Geometry: final body of the model. Coordinates: model frame, mm. A direction names the side the tool comes from. Give positions to 0.01 mm unless a question says otherwise; leave off trailing zeros. Loops run counter-clockwise (first coordinate to the right, second up) from the corner with the lowest first, then second, coordinate; pieces in that order, holes last. Notation, with made-up numbers: (-31, 77.25) -> (18, 77.25) arc R29 cw to (18, 116.25) -> close; hole circle Ø8 at (77, 48.5). An arc over 180 degrees is marked (long way). One line per item, written item: value. Start each with the question number.
Autodesk Inventor part; units mm, degrees
ref_plane "XZ Plane" through (0, 0, 0) normal (0, 1, 0) x (-1, 0, 0)
ref_plane "XY Plane" through (0, 0, 0) normal (0, 0, 1) x (1, 0, 0)
sketch "Sketch1" plane through (0, 0, 0) normal (0, 0, 1) x (1, 0, 0)
  circle A0 centre (0, 0) radius 76.2
  dimension "tubeDiameter" = 152.4
extrude "Extrusion1" add sketch "Sketch1" along normal mid plane 438.15
sketch "Sketch2" plane through (0, 0, -219.075) normal (0, 0, -1) x (-1, 0, 0)
  circle A0 centre (0, 0) radius 69.85
  dimension "d6" = 139.7
extrude "Extrusion2" cut sketch "Sketch2" against normal blind 406.4
sketch "Sketch3" plane through (0, 0, 219.075) normal (0, 0, 1) x (1, 0, 0)
  circle A0 centre (0, 0) radius 82.55
  circle A1 centre (0, 0) radius 76.2
  dimension "d9" = 165.1
extrude "Extrusion3" add sketch "Sketch3" against normal blind 25.4
sketch "Sketch4" plane through (0, 0, -219.075) normal (0, 0, -1) x (-1, 0, 0)
  circle A0 centre (0, 0) radius 76.2
  circle A1 centre (0, 0) radius 82.55
extrude "Extrusion4" add sketch "Sketch4" against normal blind 25.4
properties part number "telescopeTube" material "Nylon, molybdenum disulphide"
Item 1: Mould query, pull axis X, two halves, no side actions, for faces 4 (the face through (1, 1, 187.325)), 5 (the face through (-60.47, -46.367, 2.711)), 6 (the face through (68, 19, -219.075)). Classes: pulls with the +X half, pulls with the -X half, needs draft (parallel to the pull), parting line crosses it, or undercut.
Item 2: Access query for faces 1 (the face through (-17.895, -80.587, 206.553)), 2 (the face through (-24, -73, -193.675)), 3 (the face through (55.431, -42.503, -18.72)). Directions: +Z, -Z, +X, -X, +Y, -Y. A direction counts if a zero-diameter tool reaches every point of the face in a straight line with its end or side. Return the directions, or none.
Item 3: Ray query, line 1 along Y through (x, z) = (0, 76); line 2 along Z through (x, y) = (54.5, 26.5) (3 decimals); line 3 along Y through (x, z) = (-50.5, 145). Return the intervals inside material, ascending. Write a range as [from, to].
Item 4: Section B-B, the plane y = -54. Output: boundary loops of the cut face in (x, z) (3 decimals), then the cut area to 3 significant figures.
Item 5: Pin query (flat end, axial travel): pin 1 (12 mm diameter, centred on x = -6.5, z = 33, fed in from +Y); pin 2 (1.5 mm diameter, centred on x = 47.5, z = -141, fed in from +Y); pin 3 (1 mm diameter, centred on x = 42.5, z = -132, fed in from -Y). Return the tip coordinate at first contact, or that it passes through.
Item 6: Section A-A, the plane x = 0. Output: boundary loops of the cut face in (y, z) (3 decimals).
Item 7: Section C-C, the plane z = -185.5. Output: boundary loops of the cut face in (x, y), then the cut area to 3 significant figures.
Geometry check:
1. face 4: undercut
1. face 5: parting line crosses it
1. face 6: needs draft
2. face 1: +Z, -Z
2. face 2: none
2. face 3: -Z
3. line 1: y = [-76.2, -69.85], [69.85, 76.2]
3. line 2: z = [187.325, 219.075]
3. line 3: y = [-57.06, -48.26], [48.26, 57.06]
4. outline: (-62.438, -219.075) -> (-44.306, -219.075) -> (-44.306, 187.325) -> (44.306, 187.325) -> (44.306, -219.075) -> (62.438, -219.075) -> (62.438, -193.675) -> (53.763, -193.675) -> (53.763, 193.675) -> (62.438, 193.675) -> (62.438, 219.075) -> (-62.438, 219.075) -> (-62.438, 193.675) -> (-53.763, 193.675) -> (-53.763, -193.675) -> (-62.438, -193.675) -> close
4. area: 12,000 mm2
5. pin 1: stops at y = 76.2
5. pin 2: stops at y = 60.17
5. pin 3: stops at y = -63.58
6. outline: (-82.55, -219.075) -> (-69.85, -219.075) -> (-69.85, 187.325) -> (69.85, 187.325) -> (69.85, -219.075) -> (82.55, -219.075) -> (82.55, -193.675) -> (76.2, -193.675) -> (76.2, 193.675) -> (82.55, 193.675) -> (82.55, 219.075) -> (-82.55, 219.075) -> (-82.55, 193.675) -> (-76.2, 193.675) -> (-76.2, -193.675) -> (-82.55, -193.675) -> close
7. outline: circle Ø152.4 at (0, 0); hole circle Ø139.7 at (0, 0)
7. area: 2,910 mm2
